```python
from build123d import *

# Parameters (mm, degrees)
F0_W     = 63.5
F0_H     = 28.575
F0_W_2   = 46.736
F0_H_2   = 27.6352
F0_W_3   = 57.15
F0_H_3   = 8.128
F1_DEPTH = 3.175
F0_H_4   = 3.175
F0_W_4   = 35.814
F2_DEPTH = 56.642
F3_R     = 18.991869689
F4_R     = 17.8311640925
F5_R     = 14.9730007981
F6_R     = 5.08
F7_R     = 12.4823532344
F9_D     = 5.08
F9_DEPTH = 25.4
F9_TIP   = 1.5261859723


# Not quite as in the source:
# - a feature names something its author has since deleted; it is built from what else it names


with BuildPart() as f1:
    # F0 (on Front) → F1 (new body)
    with BuildSketch(Plane.XZ):
        with Locations((-171.45, 17.4625)):
            Rectangle(F0_W, F0_H)
        Polygon((-57.15, 0), (0, 0), (0, 40.3352), (-57.15, 40.3352), (-57.15, 12.7), align=None)
        with Locations((-80.518, 26.5176)):
            Rectangle(F0_W_2, F0_H_2)
        with Locations((-80.518, 54.1528)):
            Rectangle(F0_W_2, F0_H_2)
        Polygon((-103.886, 3.175), (-103.886, 12.7), (-103.886, 40.3352), (-103.886, 67.9704), (-139.7, 67.9704), (-139.7, 31.75), (-139.7, 3.175), align=None)
        with Locations((-28.575, 54.1528)):
            Rectangle(F0_W_3, F0_H_2)
        with Locations((-28.575, 72.0344)):
            Rectangle(F0_W_3, F0_H_3)
    extrude(amount=F1_DEPTH)

    # F0 (on Front) → F2 (join)
    with BuildSketch(Plane.XZ):
        with Locations((-171.45, 1.5875)):
            Rectangle(F0_W, F0_H_4)
        with Locations((-121.793, 1.5875)):
            Rectangle(F0_W_4, F0_H_4)
    extrude(amount=F2_DEPTH)

    # F3
    f3_edges = [f1.edges().sort_by_distance(p)[0] for p in [
        (-203.2, -1.5875, 31.75),
    ]]
    fillet(f3_edges, radius=F3_R)

    # F4
    f4_edges = [f1.edges().sort_by_distance(p)[0] for p in [
        (-139.7, -1.5875, 31.75),
    ]]
    fillet(f4_edges, radius=F4_R)

    # F5
    f5_edges = [f1.edges().sort_by_distance(p)[0] for p in [
        (-139.7, -1.5875, 67.9704),
    ]]
    fillet(f5_edges, radius=F5_R)

    # F6
    f6_edges = [f1.edges().sort_by_distance(p)[0] for p in [
        (-153.543, 0, 0),
        (-153.543, -3.175, 3.175),
    ]]
    fillet(f6_edges, radius=F6_R)

    # F7
    f7_edges = [f1.edges().sort_by_distance(p)[0] for p in [
        (-103.886, -56.642, 1.5875),
        (-203.2, -56.642, 1.5875),
    ]]
    fillet(f7_edges, radius=F7_R)

    # F9
    with Locations(Plane.XY.offset(3.175)):
        with Locations((-153.543, -26.2073233828), (-128.7145, -26.2073233828), (-178.3715, -26.2073233828)):
            Hole(F9_D / 2, depth=F9_DEPTH)
            with Locations((0, 0, -(F9_DEPTH + F9_TIP / 2))):  # 118° drill point
                Cone(0, F9_D / 2, F9_TIP, mode=Mode.SUBTRACT)

    # F10: F1 across face


with BuildPart() as f1_1:
    add(f1.part)
    add(f1.part.mirror(Plane(origin=(0, -1.5875, 38.0492), x_dir=(0, 1, 0), z_dir=(1, 0, 0))))


solid = f1_1.part
```
Geometry: final body of the model. Coordinates: model frame, mm. A direction names the side the tool comes from. Round coordinates to 2 decimals unless told otherwise and drop trailing zeros. Loops run counter-clockwise (first coordinate to the right, second up) from the corner with the lowest first, then second, coordinate; pieces in that order, holes last. Notation, with made-up numbers: (74, -37.5) -> (106, -37.5) arc R14 ccw to (106, -19.5) -> close; hole circle Ø9 at (20.25, -34). An arc over 180 degrees is marked (long way). Use one line per item in the form item = value. Start each with the question number.
1) Line query: L1, parallel to Y at x = 60, z = 60 (3 decimals); L2, parallel to Z at x = -142.5, y = -34.5 (3 decimals); L3, parallel to Z at x = 155.5, y = -5.5. Output: solid intervals per line, ascending.
2) Section D-D on x = 68. Output: boundary loops of the cut face in (y, z) (3 decimals), then the cut area to 3 significant figures.
3) Section A-A on y = -15.5. Output: boundary loops of the cut face in (x, z) (3 decimals).
4) Section B-B on x = 167. Output: boundary loops of the cut face in (y, z) (3 decimals).
5) First-contact query: P1, Ø1, axis at x = -75.5, z = 24, coming from the -Y side (3 decimals); P2, Ø6.5, axis at x = -178.37, y = -26.21, coming from the +Z side (3 decimals); P3, Ø3.5, axis at y = -2, z = 71.5, coming from the +X side; P4, Ø6.5, axis at y = -23.5, z = 7, coming from the -X side. Flat tips, straight axial feed; report the tip coordinate or a pass-through.
6) Access query for faces 5 (the flat face through (154, -31, 0)), 6 (the flat face through (-153, -32, 3.175)), 7 (the cylindrical face through (-107.445, -52.888, 1.61)). Directions: +Z, -Z, +X, -X, +Y, -Y. A direction counts if a zero-diameter tool reaches every point of the face in a straight line with its end or side. Return the directions, or none.
7) Draft query along X for faces 1 (the flat face through (-103.886, -19, 3)), 2 (the flat face through (-203.2, -19, 3)), 3 (the flat face through (103.886, -19, 3)), 4 (the flat face through (153, -32, 3.175)). Return one class per face: released by +X, released by -X, zero draft, split by the parting line, or undercut.
8) Section C-C on z = 35.5. Output: boundary loops of the cut face in (x, y) (3 decimals), then the cut area to 3 significant figures.
Response:
q1.L1 = -3.175 to 0
q1.L2 = 0 to 3.175
q1.L3 = 0 to 3.99
q2.outline = (-3.175, 12.7) -> (0, 12.7) -> (0, 67.97) -> (-3.175, 67.97) -> close
q2.area = 175 mm^2
q3.outline = (-203.2, 0) -> (-103.886, 0) -> (-103.886, 3.175) -> (-203.2, 3.175) -> close; (103.886, 0) -> (203.2, 0) -> (203.2, 3.175) -> (103.886, 3.175) -> close
q4.outline = (-56.642, 0) -> (-5.08, 0) arc R5.08 ccw to (0, 5.08) -> (0, 31.75) -> (-3.175, 31.75) -> (-3.175, 8.255) arc R5.08 cw to (-8.255, 3.175) -> (-56.642, 3.175) -> close
q5.P1 = -3.175
q5.P2 = 3.175
q5.P3 = 57.15
q5.P4 = through
q6.face_5 = -Z, +X, -X, +Y, -Y
q6.face_6 = +Z, +X, -X, -Y
q6.face_7 = +Z, -Z, -Y
q7.face_1 = undercut
q7.face_2 = released by -X
q7.face_3 = undercut
q7.face_4 = zero draft
q8.outline = (-146.592, -3.175) -> (146.592, -3.175) -> (146.592, 0) -> (-146.592, 0) -> close
q8.area = 931 mm^2
